```python
from build123d import *

# Parameters (mm, degrees)
SKETCH1_R           = 5
BOSS_EXTRUDE1_DEPTH = 3
SKETCH2_R           = 2.5
CUT_EXTRUDE1_DEPTH  = 3
CHAMFER1_SIZE       = 0.7
SKETCH3_R           = 2.3
BOSS_EXTRUDE2_DEPTH = 4
SKETCH4_R           = 2.7
BOSS_EXTRUDE3_DEPTH = 1
CHAMFER2_SIZE       = 0.4
SKETCH5_R           = 2.05
BOSS_EXTRUDE4_DEPTH = 0.65
CHAMFER3_SIZE       = 0.65
CUT_EXTRUDE2_REACH  = 38.562
SKETCH7_R           = 1.2
CUT_EXTRUDE3_DEPTH  = 5.65


with BuildPart() as part:
    # Sketch1 → Boss-Extrude1 (new body)
    with BuildSketch(Plane(origin=(0, 0, 0), x_dir=(1, 0, 0), z_dir=(0, 1, 0))):
        with Locations((-30, 0)):
            Circle(SKETCH1_R)
        with BuildLine():
            ThreePointArc((0.714285714, -4.948716593), (-4.948716593, -0.714285714), (-0.714285714, 4.948716593))
            ThreePointArc((-0.714285714, 4.948716593), (-15, 3.923048454), (-29.285714286, 4.948716593))
            ThreePointArc((-29.285714286, 4.948716593), (-26.22035527, 3.273268354), (-25, 0))
            ThreePointArc((-25, 0), (-26.726731646, -3.77964473), (-30.714285714, -4.948716593))
            ThreePointArc((-30.714285714, -4.948716593), (-15, -6.076951546), (0.714285714, -4.948716593))
        make_face()
        Circle(SKETCH1_R)
    extrude(amount=-BOSS_EXTRUDE1_DEPTH)

    # Sketch2 → Cut-Extrude1 (cut)
    with BuildSketch(Plane(origin=(0, 0, 0), x_dir=(1, 0, 0), z_dir=(0, 1, 0))):
        with Locations(Location((0, 0, 0), (0, 0, 270))):
            Circle(SKETCH2_R)
    extrude(amount=-CUT_EXTRUDE1_DEPTH, mode=Mode.SUBTRACT)

    # Chamfer1
    chamfer1_edges = [part.edges().sort_by_distance(p)[0] for p in [
        (0, 0, -2.5),
    ]]
    chamfer(chamfer1_edges, length=CHAMFER1_SIZE)

    # Sketch3 → Boss-Extrude2 (add)
    with BuildSketch(Plane(origin=(0, 0, 0), x_dir=(1, 0, 0), z_dir=(0, 1, 0))):
        with Locations(Location((-30, 0, 0), (0, 0, 270))):
            Circle(SKETCH3_R)
    extrude(amount=BOSS_EXTRUDE2_DEPTH)

    # Sketch4 → Boss-Extrude3 (add)
    with BuildSketch(Plane(origin=(0, 4, 0), x_dir=(1, 0, 0), z_dir=(0, 1, 0))):
        with Locations(Location((-30, 0, 0), (0, 0, 270))):
            Circle(SKETCH4_R)
    extrude(amount=BOSS_EXTRUDE3_DEPTH)

    # Chamfer2
    chamfer2_edges = [part.edges().sort_by_distance(p)[0] for p in [
        (-30, 4, -2.3),
    ]]
    chamfer(chamfer2_edges, length=CHAMFER2_SIZE - 0.0001)  # a hair under: the kernel refuses the full size

    # Sketch5 → Boss-Extrude4 (add)
    with BuildSketch(Plane(origin=(0, 5, 0), x_dir=(1, 0, 0), z_dir=(0, 1, 0))):
        with Locations(Location((-30, 0, 0), (0, 0, 270))):
            Circle(SKETCH5_R)
    extrude(amount=BOSS_EXTRUDE4_DEPTH)

    # Chamfer3
    chamfer3_edges = [part.edges().sort_by_distance(p)[0] for p in [
        (-30, 5, -2.05),
    ]]
    chamfer(chamfer3_edges, length=CHAMFER3_SIZE - 0.0001)  # a hair under: the kernel refuses the full size

    # Cut-Extrude2: up to this face of the body (flat: up to its plane)
    cut_extrude2_end = Plane(part.part.faces().sort_by_distance((-15.705189874, 0, 0.65316875))[0])
    # Sketch6 → Cut-Extrude2 (cut, up to the picked face)
    with BuildSketch(Plane(origin=(0, 5.65, 0), x_dir=(1, 0, 0), z_dir=(0, 1, 0)), mode=Mode.PRIVATE) as cut_extrude2_sk1:
        with BuildLine():
            ThreePointArc((-34.78558394, 1.448511772), (-34.948716593, 0.714285714), (-34.999869654, -0.036103206))
            Line((-34.999869654, -0.036103206), (-31.995452759, -0.469753431))
            ThreePointArc((-31.995452759, -0.469753431), (-32.028973803, 0.292857143), (-31.781167045, 1.014861547))
            Line((-31.781167045, 1.014861547), (-34.78558394, 1.448511772))
        make_face()
    cut_extrude2_tool1 = split(extrude(cut_extrude2_sk1.sketch, amount=-CUT_EXTRUDE2_REACH, mode=Mode.PRIVATE), bisect_by=cut_extrude2_end, keep=Keep.BOTH, mode=Mode.PRIVATE)
    # Sketch6 → Cut-Extrude2 (cut, up to the picked face)
    with BuildSketch(Plane(origin=(0, 5.65, 0), x_dir=(1, 0, 0), z_dir=(0, 1, 0)), mode=Mode.PRIVATE) as cut_extrude2_sk2:
        with BuildLine():
            Line((-28.218832955, -1.014861547), (-25.21441606, -1.448511772))
            ThreePointArc((-25.21441606, -1.448511772), (-25.053894476, -0.732147629), (-25, 0))
            ThreePointArc((-25, 0), (-25.000032587, 0.01805172), (-25.000130346, 0.036103206))
            Line((-25.000130346, 0.036103206), (-28.004547241, 0.469753431))
            ThreePointArc((-28.004547241, 0.469753431), (-27.963682471, 0.236454905), (-27.95, 0))
            ThreePointArc((-27.95, 0), (-28.018347603, -0.524932166), (-28.218832955, -1.014861547))
        make_face()
    cut_extrude2_tool2 = split(extrude(cut_extrude2_sk2.sketch, amount=-CUT_EXTRUDE2_REACH, mode=Mode.PRIVATE), bisect_by=cut_extrude2_end, keep=Keep.BOTH, mode=Mode.PRIVATE)
    # Sketch6 → Cut-Extrude2 (cut, up to the picked face)
    with BuildSketch(Plane(origin=(0, 5.65, 0), x_dir=(1, 0, 0), z_dir=(0, 1, 0)), mode=Mode.PRIVATE) as cut_extrude2_sk3:
        with BuildLine():
            ThreePointArc((-31.781167045, 1.014861547), (-32.028973803, 0.292857143), (-31.995452759, -0.469753431))
            Line((-31.995452759, -0.469753431), (-28.218832955, -1.014861547))
            ThreePointArc((-28.218832955, -1.014861547), (-28.018347603, -0.524932166), (-27.95, 0))
            ThreePointArc((-27.95, 0), (-27.963682471, 0.236454905), (-28.004547241, 0.469753431))
            Line((-28.004547241, 0.469753431), (-31.781167045, 1.014861547))
        make_face()
    cut_extrude2_tool3 = split(extrude(cut_extrude2_sk3.sketch, amount=-CUT_EXTRUDE2_REACH, mode=Mode.PRIVATE), bisect_by=cut_extrude2_end, keep=Keep.BOTH, mode=Mode.PRIVATE)
    # Sketch6 → Cut-Extrude2 (cut, up to the picked face)
    with BuildSketch(Plane(origin=(0, 5.65, 0), x_dir=(1, 0, 0), z_dir=(0, 1, 0)), mode=Mode.PRIVATE) as cut_extrude2_sk4:
        with BuildLine():
            ThreePointArc((-34.78558394, 1.448511772), (-34.948716593, 0.714285714), (-34.999869654, -0.036103206))
            Line((-34.999869654, -0.036103206), (-31.995452759, -0.469753431))
            ThreePointArc((-31.995452759, -0.469753431), (-32.028973803, 0.292857143), (-31.781167045, 1.014861547))
            Line((-31.781167045, 1.014861547), (-34.78558394, 1.448511772))
        make_face()
    cut_extrude2_tool4 = split(extrude(cut_extrude2_sk4.sketch, amount=-CUT_EXTRUDE2_REACH, mode=Mode.PRIVATE), bisect_by=cut_extrude2_end, keep=Keep.BOTH, mode=Mode.PRIVATE)
    # Sketch6 → Cut-Extrude2 (cut, up to the picked face)
    with BuildSketch(Plane(origin=(0, 5.65, 0), x_dir=(1, 0, 0), z_dir=(0, 1, 0)), mode=Mode.PRIVATE) as cut_extrude2_sk5:
        with BuildLine():
            Line((-28.218832955, -1.014861547), (-25.21441606, -1.448511772))
            ThreePointArc((-25.21441606, -1.448511772), (-25.053894476, -0.732147629), (-25, 0))
            ThreePointArc((-25, 0), (-25.000032587, 0.01805172), (-25.000130346, 0.036103206))
            Line((-25.000130346, 0.036103206), (-28.004547241, 0.469753431))
            ThreePointArc((-28.004547241, 0.469753431), (-27.963682471, 0.236454905), (-27.95, 0))
            ThreePointArc((-27.95, 0), (-28.018347603, -0.524932166), (-28.218832955, -1.014861547))
        make_face()
    cut_extrude2_tool5 = split(extrude(cut_extrude2_sk5.sketch, amount=-CUT_EXTRUDE2_REACH, mode=Mode.PRIVATE), bisect_by=cut_extrude2_end, keep=Keep.BOTH, mode=Mode.PRIVATE)
    add(cut_extrude2_tool1.solids().sort_by(Axis((-33.456178, 5.65, -0.498856), (0, -1, 0)))[0], mode=Mode.SUBTRACT)
    add(cut_extrude2_tool2.solids().sort_by(Axis((-26.543822, 5.65, 0.498856), (0, -1, 0)))[0], mode=Mode.SUBTRACT)
    add(cut_extrude2_tool3.solids().sort_by(Axis((-30, 5.65, 0), (0, -1, 0)))[0], mode=Mode.SUBTRACT)
    add(cut_extrude2_tool4.solids().sort_by(Axis((-33.456178, 5.65, -0.498856), (0, -1, 0)))[0], mode=Mode.SUBTRACT)
    add(cut_extrude2_tool5.solids().sort_by(Axis((-26.543822, 5.65, 0.498856), (0, -1, 0)))[0], mode=Mode.SUBTRACT)

    # Sketch7 → Cut-Extrude3 (cut)
    with BuildSketch(Plane(origin=(0, 5.65, 0), x_dir=(1, 0, 0), z_dir=(0, 1, 0))):
        with Locations((-30, 0)):
            Circle(SKETCH7_R)
    extrude(amount=-CUT_EXTRUDE3_DEPTH, mode=Mode.SUBTRACT)


solid = part.part
```
The model under review builds one solid part; all positions refer to its coordinate system, in mm. A direction names the side the tool comes from. Coordinates: 2 decimals unless noted, no trailing zeros. Write each loop counter-clockwise with the first axis right and the second up, starting at its lowest first coordinate (ties: lowest second). Pieces come first, ordered by that corner, then holes.
1) We need section C-C on x = -14. State the section outline as (y, z) points, then the cut area to 3 significant figures.
2) Clearance check with flat-ended pins moving along their axes: pin 1 Ø4 at (x, y) = (-26, 2.5) entering from +Z; pin 2 Ø3.5 at (x, z) = (-19.5, -0.5) entering from +Y; pin 3 Ø6 at (x, z) = (-30, 1) entering from +Y. State where each tip first meets the part, or that it passes through.
3) We need section D-D on x = -9. State the section outline as (y, z) points.
4) Machinability: for faces 5 (the face through (-29.63, 1.77, -2.27)), 6 (the face through (-2.44, -1.83, -0.54)), 7 (the face through (-30.39, 3.71, 2.38)), 8 (the face through (-30.186, 2.865, 1.185)), which of the approach directions +Z, -Z, +X, -X, +Y, -Y give a long, thin tool a straight path to every point of the face, cutting with its end or side? Answer none if there is none.
5) We need section B-B on x = 0. State the section outline as (y, z) points.
6) The part is to be moulded in two halves that separate along Z. For faces 1 (the face through (-30.37, 1.77, 2.27)), 2 (the face through (-29.566, 4.493, -2.665)), 3 (the face through (-30.1, 5.65, 1.4)), 4 (the face through (-29.814, 2.865, -1.185)), say which applies: pulls with the +Z half, pulls with the -Z half, needs draft (parallel to the pull), parting line crosses it, or undercut.
7) We need section A-A on y = 0.75. State the section outline as (x, z) points, then the cut area to 3 significant figures.
8) To check wall thickness, follow probe 1 along X at (y, z) = (-1.3, 0); probe 2 along Y at (x, z) = (-20, 1); probe 3 along Y at (x, z) = (-30.5, -2.5). State the ranges of each line that lie inside material, in increasing order.
Answer list:
1. outline: (-3, -3.93) - (0, -3.93) - (0, 6.07) - (-3, 6.07) - close
1. area: 30.0 mm2
2. pin 1: stops at z = 1.14
2. pin 2: stops at y = 0
2. pin 3: stops at y = 5.65
3. outline: (-3, -4.1) - (0, -4.1) - (0, 5.91) - (-3, 5.91) - close
4. face 5: -Z
4. face 6: +Y, -Y
4. face 7: +Z
4. face 8: +Y
5. outline: (-3, -5) - (0, -5) - (0, -3.2) - (-0.7, -2.5) - (-3, -2.5) - close; (-3, 2.5) - (-0.7, 2.5) - (0, 3.2) - (0, 5.05) - (-3, 5.05) - close
6. face 1: pulls with the +Z half
6. face 2: pulls with the -Z half
6. face 3: needs draft
6. face 4: undercut
7. outline: (-32.26, 0.43) - (-31.03, 0.61) arc R1.2 cw to (-29.18, 0.88) - (-27.96, 1.05) arc R2.3 ccw to start; (-32.04, -1.05) arc R2.3 ccw to (-27.74, -0.43) - (-28.97, -0.61) arc R1.2 cw to (-30.82, -0.88) - close
7. area: 8.67 mm2
8. probe 1: x = -35 to -2.5, 2.5 to 5
8. probe 2: y = -3 to 0
8. probe 3: y = -3 to 0, 3.85 to 5.15
